Geometry check sheet. Reference: drawing and pictorial views, mm from the part's lowest x, y, z. A direction names the side the tool comes from. Round coordinates to 2 decimals unless told otherwise and drop trailing zeros. Order: outer loops, then holes, each group sorted by start corner. A loop starts at its lowest first (then second) coordinate and runs counter-clockwise, first axis right, second up. Notation, with made-up numbers: (77, -27.5) -> (94, -27.5) arc R25 ccw to (94, 1.5) -> close; hole circle Ø10 at (7.5, 53.25). An arc over 180 degrees is marked (long way). Return JSON: item names as keys, results as strings. Group by question number.
1) Section check A-A on y = 38.5. Enter the section's corners in (x, z).
2) Scan lines: L1, parallel to Z at x = 130, y = 1; L2, parallel to X at y = 2.2, z = 90; L3, parallel to X at y = 45.5, z = 26.5. Record each from-to range of solid material in increasing order.
3) Section check C-C on z = 43. Enter the section's corners in (x, y).
4) Tool access check on the marked faces 1 and 2. Record the directions out of +Z, -Z, +X, -X, +Y, -Y that give a thin tool (end or side, any length) a straight path to the whole face; none if there is none.
5) Draft check along X on the marked faces 3, 4 and 5. Enter one of: pulls with the +X half, pulls with the -X half, needs draft (parallel to the pull), parting line crosses it, or undercut.
6) Depth check by flat-ended pin: pin 1 (5 mm diameter, centred on x = 95.5, z = 47, fed in from +Y); pin 2 (2.5 mm diameter, centred on x = 130, z = 20, fed in from -Y). Enter the tip coordinate at first touch or a pass-through.
7) Section check B-B on x = 46.5. Enter the section's corners in (y, z).
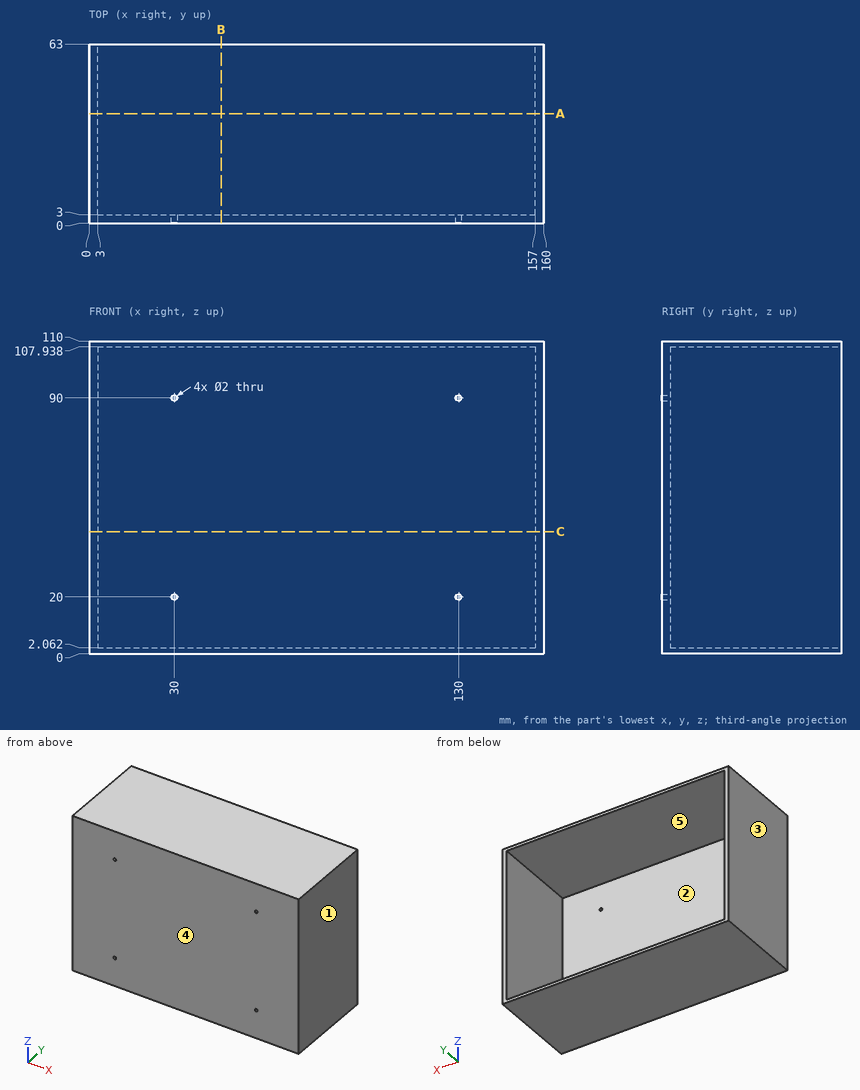
Check result:
{
 "1": {"outline": "(0, 0) -> (160, 0) -> (160, 110) -> (0, 110) -> close; hole (3, 2.06) -> (157, 2.06) -> (157, 107.94) -> (3, 107.94) -> close"},
 "2": {"L1": "0 to 19, 21 to 89, 91 to 110", "L2": "0 to 29, 31 to 129, 131 to 160", "L3": "0 to 3, 157 to 160"},
 "3": {"outline": "(0, 0) -> (160, 0) -> (160, 63) -> (157, 63) -> (157, 3) -> (3, 3) -> (3, 63) -> (0, 63) -> close"},
 "4": {"face 1": "+Z, -Z, +X, +Y, -Y", "face 2": "+Y"},
 "5": {"face 3": "pulls with the -X half", "face 4": "needs draft", "face 5": "undercut"},
 "6": {"pin 1": "y = 3", "pin 2": "y = 0"},
 "7": {"outline": "(0, 0) -> (63, 0) -> (63, 2.06) -> (3, 2.06) -> (3, 107.94) -> (63, 107.94) -> (63, 110) -> (0, 110) -> close"}
}
